Here's the drawing with two shaded views (mm, measured from the low corner). I have some questions. A direction names the side the tool comes from. Give positions to 0.01 mm unless a question says otherwise; leave off trailing zeros. Write each loop counter-clockwise with the first axis right and the second up, starting at its lowest first coordinate (ties: lowest second). Pieces come first, ordered by that corner, then holes. Notation, with made-up numbers: (54.5, -8.5) - (59.5, -8.5) arc R13 ccw to (59.5, 14.5) - close; hole circle Ø11 at (57.25, -26.75). An arc over 180 degrees is marked (long way). Write item = value, one per line.
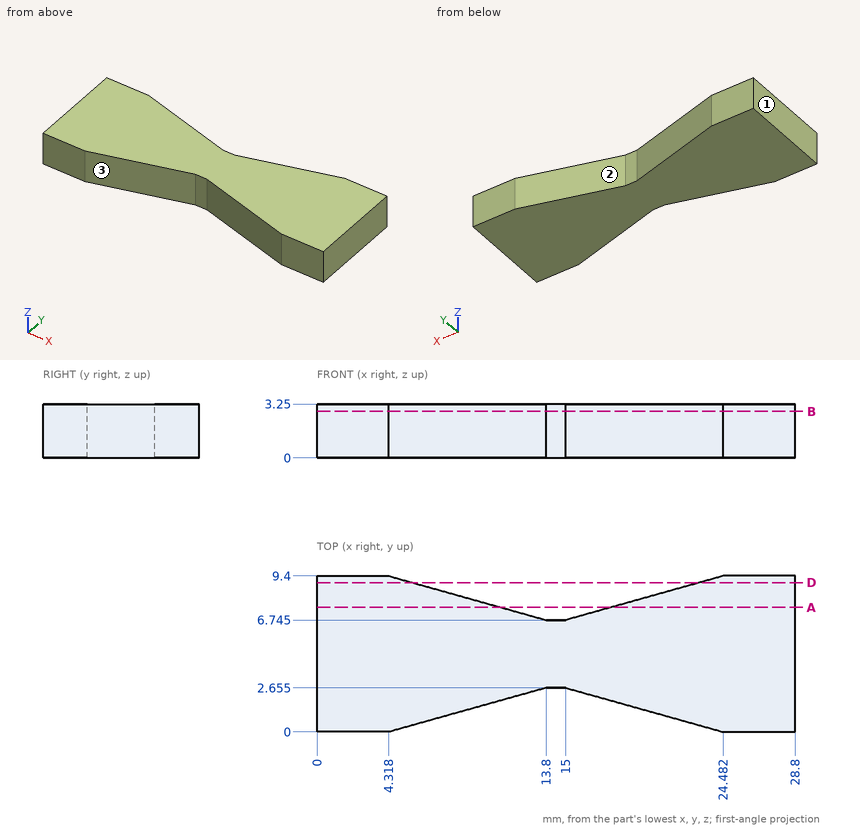
1. I need wall thicknesses on line 1 (Y direction, x = 14.75, z = 2.2) (1 decimal); line 2 (Y direction, x = 19, z = 0.4) (1 decimal). Which ranges of each line are inside material? Lowest first, please.
Filled sheet:
line_1 = 2.7 to 6.7
line_2 = 1.5 to 7.9
2. Which directions (+Z, -Z, +X, -X, +Y, -Y) give clear straight access to the entire face, cutting with the end or side of a thin tool? Please do the marked faces 1, 2 and 3.
Filled sheet:
face_1 = +Z, -Z, -X, +Y, -Y
face_2 = +Z, -Z, +Y
face_3 = +Z, -Z, -Y
3. For pin 1 (1.3 mm diameter, centred on x = 14.5, z = 1.5, fed in from -Y), with a flat end and sliding along its axis, tell me the tip position at first contact or that it passes through.
Filled sheet:
pin_1 = 2.61
4. If we section it at B-B, the plane z = 2.8: Please give me the cut outline in (x, y) (1 decimal).
Filled sheet:
outline = (0, 0) - (4.3, 0) - (13.8, 2.7) - (15, 2.7) - (24.5, 0) - (28.8, 0) - (28.8, 9.4) - (24.5, 9.4) - (15, 6.7) - (13.8, 6.7) - (4.3, 9.4) - (0, 9.4) - close
5. If we section it at D-D, the plane y = 9: Please give me the cut outline in (x, z).
Filled sheet:
outline = (0, 0) - (5.75, 0) - (5.75, 3.25) - (0, 3.25) - close; (23.05, 0) - (28.8, 0) - (28.8, 3.25) - (23.05, 3.25) - close
6. If we section it at A-A, the plane y = 7.5: Please give me the cut outline in (x, z).
Filled sheet:
outline = (0, 0) - (11.1, 0) - (11.1, 3.25) - (0, 3.25) - close; (17.7, 0) - (28.8, 0) - (28.8, 3.25) - (17.7, 3.25) - close
